from build123d import *

# Parameters (mm, degrees)
SKETCH1_W           = 44.958
SKETCH1_H           = 67.818
BOSS_EXTRUDE1_DEPTH = 90.17
SKETCH2_R           = 5
CUT_EXTRUDE1_DEPTH  = 6.35
SKETCH3_R           = 4.064
CUT_EXTRUDE2_DEPTH  = 68.818
SKETCH4_R           = 5.1
CUT_EXTRUDE3_DEPTH  = 15.24
SKETCH5_R           = 5.08
CUT_EXTRUDE4_DEPTH  = 50.8
SKETCH6_W           = 24.13
SKETCH6_H           = 19.05
CUT_EXTRUDE5_DEPTH  = 34.29
FILLET1_R           = 3.81


with BuildPart() as part:
    # Sketch1 → Boss-Extrude1 (new body)
    with BuildSketch(Plane.XY):
        with Locations((22.479, 33.909)):
            Rectangle(SKETCH1_W, SKETCH1_H)
    extrude(amount=BOSS_EXTRUDE1_DEPTH)

    # Sketch2 → Cut-Extrude1 (cut)
    with BuildSketch(Plane(origin=(44.958, 0, 0), x_dir=(0, 0, -1), z_dir=(1, 0, 0))):
        with Locations((-44.45, 50.66)):
            Circle(SKETCH2_R)
        with Locations((-44.45, 10.16)):
            Circle(SKETCH2_R)
    extrude(amount=-CUT_EXTRUDE1_DEPTH, mode=Mode.SUBTRACT)

    # Sketch3 → Cut-Extrude2 (cut, through all)
    with BuildSketch(Plane(origin=(0, 67.818, 0), x_dir=(1, 0, 0), z_dir=(0, 1, 0))):
        with Locations((22.479, -19.05)):
            Circle(SKETCH3_R)
    extrude(amount=-CUT_EXTRUDE2_DEPTH, mode=Mode.SUBTRACT)

    # Sketch4 → Cut-Extrude3 (cut)
    with BuildSketch(Plane(origin=(0, 67.818, 0), x_dir=(1, 0, 0), z_dir=(0, 1, 0))):
        with Locations((22.479, -19.05)):
            Circle(SKETCH4_R)
    extrude(amount=-CUT_EXTRUDE3_DEPTH, mode=Mode.SUBTRACT)

    # Sketch5 → Cut-Extrude4 (cut)
    with BuildSketch(Plane.XY.offset(90.17)):
        with Locations((22.479, 34.036)):
            Circle(SKETCH5_R)
    extrude(amount=-CUT_EXTRUDE4_DEPTH, mode=Mode.SUBTRACT)

    # Sketch6 → Cut-Extrude5 (cut)
    with BuildSketch(Plane(origin=(44.958, 0, 0), x_dir=(0, 0, -1), z_dir=(1, 0, 0))):
        with Locations((-46.355, 33.909)):
            Rectangle(SKETCH6_W, SKETCH6_H)
    extrude(amount=-CUT_EXTRUDE5_DEPTH, mode=Mode.SUBTRACT)

    # Fillet1
    fillet1_edges = [part.edges().sort_by_distance(p)[0] for p in [
        (44.958, 33.909, 90.17),
        (0, 33.909, 90.17),
        (44.958, 33.909, 0),
        (0, 33.909, 0),
    ]]
    fillet(fillet1_edges, radius=FILLET1_R)


solid = part.part
Geometry: final body of the model. Coordinates: model frame, mm. A direction names the side the tool comes from. Give positions to 0.01 mm unless a question says otherwise; leave off trailing zeros. Write each loop counter-clockwise with the first axis right and the second up, starting at its lowest first coordinate (ties: lowest second). Pieces come first, ordered by that corner, then holes. Notation, with made-up numbers: (8, 44) -> (15, 44) arc R23 ccw to (15, 78) -> close; hole circle Ø7 at (54, 39). An arc over 180 degrees is marked (long way). Answer as a JSON object with one key per item and string values.
1. Contact query for a flat-ended pin moving along its axis: pin 1 (9 mm diameter, centred on y = 50.66, z = 44.45, fed in from +X). Output: stop coordinate, or through.
Ans:
{"pin 1": "stops at x = 38.61"}
2. Access query for faces 4 (the cylindrical face through (1.086, 34.384, 89.024)), 5 (the flat face through (22, 34, 0)), 6 (the cylindrical face through (27.324, 35.562, 74.517)), 7 (the flat face through (21, 52.578, 23)), 8 (the flat face through (38.608, 10, 45)). Directions: +Z, -Z, +X, -X, +Y, -Y. A direction counts if a zero-diameter tool reaches every point of the face in a straight line with its end or side. Return the directions, or none.
Ans:
{"face 4": "+Z, -X, +Y, -Y", "face 5": "-Z, +X, -X, +Y, -Y", "face 6": "+Z", "face 7": "+Y", "face 8": "+X"}
3. Cut plane D-D on z = 44.45. Output: boundary loops of the cut face in (x, y), and give its area (3 significant figures).
Ans:
{"outline": "(0, 0) -> (44.96, 0) -> (44.96, 5.16) -> (38.61, 5.16) -> (38.61, 15.16) -> (44.96, 15.16) -> (44.96, 24.38) -> (10.67, 24.38) -> (10.67, 43.43) -> (44.96, 43.43) -> (44.96, 45.66) -> (38.61, 45.66) -> (38.61, 55.66) -> (44.96, 55.66) -> (44.96, 67.82) -> (0, 67.82) -> close", "area": "2,270 mm^2"}
4. Cut plane C-C on x = 29. Output: boundary loops of the cut face in (y, z), and give its area (3 significant figures).
Ans:
{"outline": "(0, 0) -> (67.82, 0) -> (67.82, 90.17) -> (0, 90.17) -> close; hole (24.38, 34.29) -> (43.43, 34.29) -> (43.43, 58.42) -> (24.38, 58.42) -> close", "area": "5,660 mm^2"}
5. Cut plane B-B on y = 10.16. Output: boundary loops of the cut face in (x, z).
Ans:
{"outline": "(0, 3.81) arc R3.81 ccw to (3.81, 0) -> (41.15, 0) arc R3.81 ccw to (44.96, 3.81) -> (44.96, 39.45) -> (38.61, 39.45) -> (38.61, 49.45) -> (44.96, 49.45) -> (44.96, 86.36) arc R3.81 ccw to (41.15, 90.17) -> (3.81, 90.17) arc R3.81 ccw to (0, 86.36) -> close; hole circle Ø8.13 at (22.48, 19.05)"}
6. Mould query, pull axis Z, two halves, no side actions, for faces 1 (the cylindrical face through (43.812, 34.384, 89.084)), 2 (the flat face through (28, 34, 34.29)), 3 (the flat face through (44.958, 18, 45)). Classes: pulls with the +Z half, pulls with the -Z half, needs draft (parallel to the pull), parting line crosses it, or undercut.
Ans:
{"face 1": "pulls with the +Z half", "face 2": "undercut", "face 3": "needs draft"}
7. Ray query, probe 1 along Y at (x, z) = (41.5, 44.45); probe 2 along Y at (x, z) = (21.5, 54); probe 3 along Y at (x, z) = (42, 44). Return the intervals inside material, ascending. Write a range as from..to.
Ans:
{"probe 1": "y = 0..5.16, 15.16..24.38, 43.43..45.66, 55.66..67.82", "probe 2": "y = 0..24.38, 43.43..67.82", "probe 3": "y = 0..5.18, 15.14..24.38, 43.43..45.68, 55.64..67.82"}
8. Cut plane A-A on z = 19.05. Output: boundary loops of the cut face in (x, y) (3 decimals), and give its area (3 significant figures).
Ans:
{"outline": "(0, 0) -> (18.415, 0) -> (18.415, 52.578) -> (17.379, 52.578) -> (17.379, 67.818) -> (0, 67.818) -> close; (26.543, 0) -> (44.958, 0) -> (44.958, 67.818) -> (27.579, 67.818) -> (27.579, 52.578) -> (26.543, 52.578) -> close", "area": "2,470 mm^2"}
